Part print with two shaded views. Sizes in mm from the minimum x, y, z corner. A direction names the side the tool comes from. Coordinates: 2 decimals unless noted, no trailing zeros. Loops run counter-clockwise (first coordinate to the right, second up) from the corner with the lowest first, then second, coordinate; pieces in that order, holes last. Notation, with made-up numbers: (60, 23.25) -> (106, 23.25) arc R26 ccw to (106, 37.25) -> close; hole circle Ø4 at (46.5, 8). An arc over 180 degrees is marked (long way). Return JSON: item names as keys, results as strings. Group by question number.
(1) Probe L1, parallel to X at y = 26.5, z = 56.5; L2, parallel to X at y = 48.5, z = 112. List the from-to ranges inside material, lowest first.
(2) Tool access for the marked faces 4, 5, 6, 7 and 8: list every direction of +Z, -Z, +X, -X, +Y, -Y with a clear straight run to the whole face (end or side of a thin tool).
(3) Flat gauge pins, fed straight in: pin 1 Ø4 at (x, y) = (42.5, 20) entering from +Z; pin 2 Ø6 at (x, y) = (60, 34.5) entering from +Z; pin 3 Ø1 at (y, z) = (62, 120.5) entering from -X. Where does each tip first touch, or does it go through?
(4) Mould opens along Z. For the marked faces 1, 2 and 3 say: pulls with the +Z half, pulls with the -Z half, needs draft (parallel to the pull), parting line crosses it, or undercut.
(5) Saw through at B-B on x = 38.1. Write the cut outline in (y, z), then the cut area to 3 significant figures.
(6) Saw through at C-C on y = 30. Write the cut outline in (x, z).
(7) Saw through at A-A on z = 38.1. Write the cut outline in (x, y), then the cut area to 3 significant figures.
(8) Saw through at D-D on x = 73.5. Write the cut outline in (y, z), then the cut area to 3 significant figures.
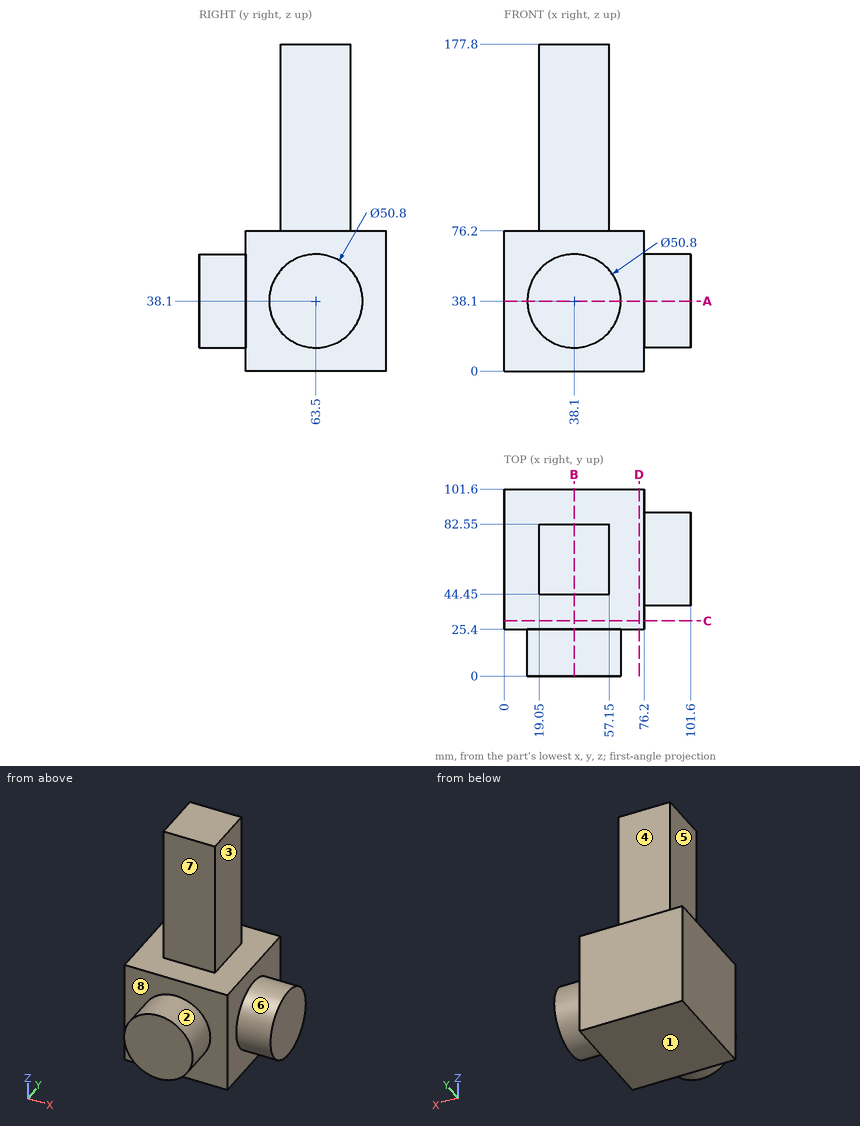
Geometry results:
{
 "1": {"L1": "0 to 76.2", "L2": "19.05 to 57.15"},
 "2": {"face 4": "+Z, +X, -X, +Y", "face 5": "+Z, -X, +Y, -Y", "face 6": "+X", "face 7": "+Z, +X, -X, -Y", "face 8": "-Y"},
 "3": {"pin 1": "z = 63.39", "pin 2": "z = 76.2", "pin 3": "x = 19.05"},
 "4": {"face 1": "pulls with the -Z half", "face 2": "parting line crosses it", "face 3": "needs draft"},
 "5": {"outline": "(0, 12.7) -> (25.4, 12.7) -> (25.4, 0) -> (101.6, 0) -> (101.6, 76.2) -> (82.55, 76.2) -> (82.55, 177.8) -> (44.45, 177.8) -> (44.45, 76.2) -> (25.4, 76.2) -> (25.4, 63.5) -> (0, 63.5) -> close", "area": "11,000 mm²"},
 "6": {"outline": "(0, 0) -> (76.2, 0) -> (76.2, 76.2) -> (0, 76.2) -> close"},
 "7": {"outline": "(0, 25.4) -> (12.7, 25.4) -> (12.7, 0) -> (63.5, 0) -> (63.5, 25.4) -> (76.2, 25.4) -> (76.2, 38.1) -> (101.6, 38.1) -> (101.6, 88.9) -> (76.2, 88.9) -> (76.2, 101.6) -> (0, 101.6) -> close", "area": "8,390 mm²"},
 "8": {"outline": "(25.4, 0) -> (101.6, 0) -> (101.6, 76.2) -> (25.4, 76.2) -> close", "area": "5,810 mm²"}
}
